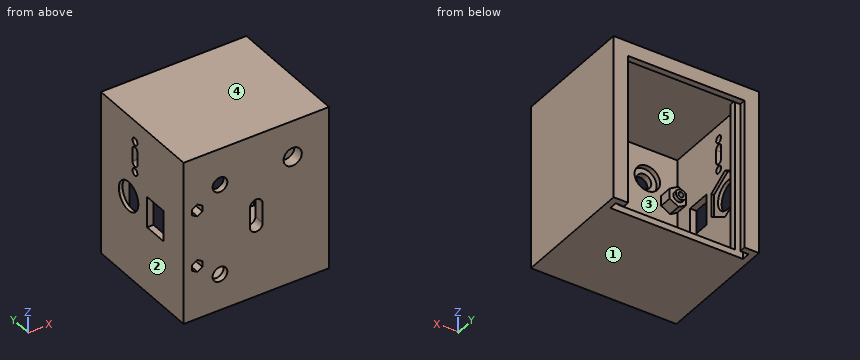
from build123d import *

# Parameters (mm, degrees)
SKETCH1_W               = 80
SKETCH1_H               = 90
BOSS_EXTRUDE1_DEPTH     = 6
SKETCH4_W               = 80
SKETCH4_H               = 90
SKETCH4_W_2             = 73
SKETCH4_H_2             = 83
BOSS_EXTRUDE2_DEPTH     = 54
SKETCH6_R               = 4.05
SKETCH6_R_2             = 5
CUT_EXTRUDE1_DEPTH      = 40
SKETCH7_R               = 7
CUT_EXTRUDE2_DEPTH      = 2.8
BOSS_EXTRUDE3_DEPTH     = 7
SKETCH11_R              = 2.85
BOSS_EXTRUDE4_DEPTH     = 2
CUT_EXTRUDE3_DEPTH      = 9
CUT_EXTRUDE3_DEPTH_BACK = 6
SKETCH5_R               = 1.5
CUT_EXTRUDE4_DEPTH      = 6
CUT_EXTRUDE4_DEPTH_BACK = 81.876448982
SKETCH12_W              = 17
SKETCH12_H              = 13.5
CUT_EXTRUDE6_DEPTH      = 3.5
SKETCH17_R              = 8
CUT_EXTRUDE8_DEPTH      = 2
CUT_EXTRUDE9_DEPTH      = 1.5
CUT_EXTRUDE10_DEPTH     = 10
BOSS_EXTRUDE5_DEPTH     = 90
BOSS_EXTRUDE5_2_DEPTH   = 90
SKETCH21_W              = 3.5
SKETCH21_H              = 8
BOSS_EXTRUDE6_DEPTH     = 80
SKETCH22_W              = 80
SKETCH22_H              = 3.5
BOSS_EXTRUDE7_DEPTH     = 4.5
SKETCH24_W              = 8
SKETCH24_H              = 3.5
BOSS_EXTRUDE8_DEPTH     = 90
SKETCH26_R              = 2
CUT_EXTRUDE11_DEPTH     = 3.5


with BuildPart() as part:
    # Sketch1 → Boss-Extrude1 (new body)
    with BuildSketch(Plane(origin=(0, 0, 0), x_dir=(1, 0, 0), z_dir=(0, 1, 0))):
        Rectangle(SKETCH1_W, SKETCH1_H)
    extrude(amount=BOSS_EXTRUDE1_DEPTH)

    # Sketch4 → Boss-Extrude2 (add)
    with BuildSketch(Plane(origin=(0, 6, 0), x_dir=(1, 0, 0), z_dir=(0, 1, 0))):
        Rectangle(SKETCH4_W, SKETCH4_H)
        Rectangle(SKETCH4_W_2, SKETCH4_H_2, mode=Mode.SUBTRACT)
    extrude(amount=BOSS_EXTRUDE2_DEPTH)

    # Sketch6 → Cut-Extrude1 (cut)
    with BuildSketch(Plane(origin=(0, 6, 0), x_dir=(1, 0, 0), z_dir=(0, 1, 0))):
        with Locations(Location((-20, 25, 0), (0, 0, 270))):
            Circle(SKETCH6_R)
        with Locations(Location((-20, -25, 0), (0, 0, 270))):
            Circle(SKETCH6_R)
        with Locations(Location((20, -25, 0), (0, 0, 270))):
            Circle(SKETCH6_R_2)
    extrude(amount=-CUT_EXTRUDE1_DEPTH, mode=Mode.SUBTRACT)

    # Sketch7 → Cut-Extrude2 (cut)
    with BuildSketch(Plane(origin=(0, 6, 0), x_dir=(1, 0, 0), z_dir=(0, 1, 0))):
        with Locations(Location((-20, 25, 0), (0, 0, 270))):
            Circle(SKETCH7_R)
        with Locations(Location((-20, -25, 0), (0, 0, 270))):
            Circle(SKETCH7_R)
    extrude(amount=-CUT_EXTRUDE2_DEPTH, mode=Mode.SUBTRACT)

    # Sketch10 → Boss-Extrude3 (add)
    with BuildSketch(Plane(origin=(0, 6, 0), x_dir=(1, 0, 0), z_dir=(0, 1, 0))):
        Polygon((-32.5, 21.100297611), (-37.35, 18.300148806), (-37.35, 12.699851194), (-32.5, 9.899702389), (-27.65, 12.699851194), (-27.65, 18.300148806), align=None)
        Polygon((-27.65, -12.699851194), (-32.5, -9.899702389), (-37.35, -12.699851194), (-37.35, -18.300148806), (-32.5, -21.100297611), (-27.65, -18.300148806), align=None)
    extrude(amount=BOSS_EXTRUDE3_DEPTH)

    # Sketch11 → Boss-Extrude4 (add)
    with BuildSketch(Plane(origin=(0, 13, 0), x_dir=(1, 0, 0), z_dir=(0, 1, 0))):
        with Locations(Location((-32.5, 15.5, 0), (0, 0, 270))):
            Circle(SKETCH11_R)
        with Locations(Location((-32.5, -15.5, 0), (0, 0, 270))):
            Circle(SKETCH11_R)
    extrude(amount=BOSS_EXTRUDE4_DEPTH)

    # Sketch5 → Cut-Extrude3 (cut, two sides: drawn at the far end of the back side and taken through both)
    with BuildSketch(Plane(origin=(0, 6, 0), x_dir=(1, 0, 0), z_dir=(0, 1, 0)).offset(-CUT_EXTRUDE3_DEPTH_BACK)):
        with Locations(Location((-32.5, 15.5, 0), (0, 0, 270))):
            Circle(SKETCH5_R)
        with Locations(Location((-32.5, -15.5, 0), (0, 0, 270))):
            Circle(SKETCH5_R)
    extrude(amount=CUT_EXTRUDE3_DEPTH + CUT_EXTRUDE3_DEPTH_BACK, mode=Mode.SUBTRACT)

    # Sketch8 → Cut-Extrude4 (cut, two sides: drawn at the far end of the back side and taken through both)
    with BuildSketch(Plane(origin=(0, 6, 0), x_dir=(1, 0, 0), z_dir=(0, 1, 0)).offset(-CUT_EXTRUDE4_DEPTH_BACK)):
        Polygon((-29.65, 17.145448267), (-32.5, 18.790896534), (-35.35, 17.145448267), (-35.35, 13.854551733), (-32.5, 12.209103466), (-29.65, 13.854551733), align=None)
        Polygon((-29.65, -13.854551733), (-32.5, -12.209103466), (-35.35, -13.854551733), (-35.35, -17.145448267), (-32.5, -18.790896534), (-29.65, -17.145448267), align=None)
    extrude(amount=CUT_EXTRUDE4_DEPTH + CUT_EXTRUDE4_DEPTH_BACK, mode=Mode.SUBTRACT)

    # Sketch12 → Cut-Extrude6 (cut)
    with BuildSketch(Plane(origin=(-36.5, 0, 0), x_dir=(0, 0, -1), z_dir=(1, 0, 0))):
        with Locations((0, 23.25)):
            Rectangle(SKETCH12_W, SKETCH12_H)
    extrude(amount=-CUT_EXTRUDE6_DEPTH, mode=Mode.SUBTRACT)

    # Sketch17 → Cut-Extrude8 (cut)
    with BuildSketch(Plane.ZY.offset(40)):
        with Locations((0, 45.25)):
            Circle(SKETCH17_R)
    extrude(amount=-CUT_EXTRUDE8_DEPTH, mode=Mode.SUBTRACT)

    # Sketch15 → Cut-Extrude9 (cut)
    with BuildSketch(Plane(origin=(-36.5, 0, 0), x_dir=(0, 0, -1), z_dir=(1, 0, 0))):
        Polygon((-6.495190528, 56.5), (-12.990381057, 45.25), (-6.495190528, 34), (6.495190528, 34), (12.990381057, 45.25), (6.495190528, 56.5), align=None)
    extrude(amount=-CUT_EXTRUDE9_DEPTH, mode=Mode.SUBTRACT)

    # Sketch19 → Cut-Extrude10 (cut)
    with BuildSketch(Plane(origin=(0, 6, 0), x_dir=(1, 0, 0), z_dir=(0, 1, 0))):
        with BuildLine():
            Line((-3.5, -5.5), (-3.5, 5.5))
            ThreePointArc((-3.5, 5.5), (0, 9), (3.5, 5.5))
            Line((3.5, 5.5), (3.5, -5.5))
            ThreePointArc((3.5, -5.5), (0, -9), (-3.5, -5.5))
        make_face()
    extrude(amount=-CUT_EXTRUDE10_DEPTH, mode=Mode.SUBTRACT)



with BuildPart() as body_2:
    # Sketch20 → Boss-Extrude5 (new body)
    with BuildSketch(Plane(origin=(0, 0, -45), x_dir=(-1, 0, 0), z_dir=(0, 0, -1))):
        Polygon((-40, 60), (-36.5, 60), (-36.5, 64.5), (-32, 64.5), (-32, 68), (-40, 68), align=None)
    extrude(amount=-BOSS_EXTRUDE5_DEPTH)


with BuildPart() as body_3:
    # Sketch20 → Boss-Extrude5 2 (new body)
    with BuildSketch(Plane(origin=(0, 0, -45), x_dir=(-1, 0, 0), z_dir=(0, 0, -1))):
        Polygon((40, 60), (36.5, 60), (36.5, 64.5), (32, 64.5), (32, 68), (40, 68), align=None)
    extrude(amount=-BOSS_EXTRUDE5_2_DEPTH)


with BuildPart() as part_1:
    add(part.part)

    add(body_2.part)  # Boss-Extrude6 merges body 2
    # Sketch21 → Boss-Extrude6 (add)
    with BuildSketch(Plane(origin=(40, 0, 0), x_dir=(0, 0, -1), z_dir=(1, 0, 0))):
        with Locations((-43.25, 64)):
            Rectangle(SKETCH21_W, SKETCH21_H)
    extrude(amount=-BOSS_EXTRUDE6_DEPTH)


    add(body_3.part)  # Boss-Extrude7 merges body 3
    # Sketch22 → Boss-Extrude7 (add)
    with BuildSketch(Plane(origin=(0, 0, 41.5), x_dir=(-1, 0, 0), z_dir=(0, 0, -1))):
        with Locations((0, 66.25)):
            Rectangle(SKETCH22_W, SKETCH22_H)
    extrude(amount=BOSS_EXTRUDE7_DEPTH)

    # Sketch24 → Boss-Extrude8 (add)
    with BuildSketch(Plane.XY.offset(45)):
        with Locations((-36, 58.25)):
            Rectangle(SKETCH24_W, SKETCH24_H)
        with Locations((36, 58.25)):
            Rectangle(SKETCH24_W, SKETCH24_H)
    extrude(amount=-BOSS_EXTRUDE8_DEPTH)

    # Sketch26 → Cut-Extrude11 (cut)
    with BuildSketch(Plane.ZY.offset(40)):
        with Locations((16.5, 40)):
            Circle(SKETCH26_R)
        with Locations((33.5, 40)):
            Circle(SKETCH26_R)
        with BuildLine():
            Line((21.5, 42), (28.5, 42))
            ThreePointArc((28.5, 42), (30.5, 40), (28.5, 38))
            Line((28.5, 38), (21.5, 38))
            ThreePointArc((21.5, 38), (19.5, 40), (21.5, 42))
        make_face()
    extrude(amount=-CUT_EXTRUDE11_DEPTH, mode=Mode.SUBTRACT)


solid = part_1.part
Can you work these out from the model? Positions are in its coordinate system, mm. Face numbers are marked on the shaded views. A direction names the side the tool comes from. Give positions to 0.01 mm unless a question says otherwise; leave off trailing zeros. Write each loop counter-clockwise with the first axis right and the second up, starting at its lowest first coordinate (ties: lowest second). Pieces come first, ordered by that corner, then holes. Notation, with made-up numbers: M 20,-19 L 33,-19 A35 cw 33,13 Z; hole C 11,-14 d11. An arc over 180 degrees is marked long. Answer in a Markdown table with one row per item. Add a question column.
Item 1: Imagine slicing it at C-C, the plane y = 10.5. State how many separate pieces and enclosed holes the cut face has, plus the area to 3 significant figures.
Item 2: We'd pull the mould along X, two halves only. Please class the marked faces 1, 2 and 3: released by +X, released by -X, zero draft, split by the parting line, or undercut.
Item 3: Please list where these lines run through material, in increasing order: L1, parallel to X at y = 12.8, z = -15.5; L2, parallel to X at y = 2.45, z = 25; L3, parallel to Z at x = -23, y = 38.
Item 4: Imagine slicing it at D-D, the plane x = 0. Write out the boundary of the cut face in (y, z), plus the area to 3 significant figures.
Item 5: For pin 1 Ø5 at (x, z) = (25.5, 2) entering from +Y; pin 2 Ø3 at (x, z) = (-21.5, 24) entering from +Y; pin 3 Ø3.5 at (y, z) = (40, 16.5) entering from -X, each with a flat end and sliding along its axis, tell me the tip position at first contact or that it passes through.
Item 6: Imagine slicing it at A-A, the plane x = -20. Write out the boundary of the cut face in (y, z), plus the area to 3 significant figures.
Item 7: On a 3-axis mill with a long thin cutter (end or side, diameter ignored), from which of +Z, -Z, +X, -X, +Y, -Y can I reach the whole of each face in a straight line? I mean the marked faces 4 and 5. Say none if no direction works.
Evaluation:
| question | item | result |
|---|---|---|
| 1 | separate pieces | 1 |
| 1 | enclosed holes | 3 |
| 1 | area | 1,240 mm² |
| 2 | face 1 | zero draft |
| 2 | face 2 | released by -X |
| 2 | face 3 | undercut |
| 3 | L1 | x = -40 to -34, -31 to -27.65, 36.5 to 40 |
| 3 | L2 | x = -40 to -24.05, -15.95 to 15, 25 to 40 |
| 3 | L3 | z = -45 to -41.5, 41.5 to 45 |
| 4 | outline | M 0,-45 L 60,-45 L 60,-41.5 L 6,-41.5 L 6,-9 L 0,-9 Z; M 0,9 L 6,9 L 6,41.5 L 64.5,41.5 L 64.5,37 L 68,37 L 68,45 L 0,45 Z |
| 4 | area | 854 mm² |
| 5 | pin 1 | stops at y = 6 |
| 5 | pin 2 | passes through |
| 5 | pin 3 | stops at x = 36.5 |
| 6 | outline | M 0,-45 L 60,-45 L 60,-41.5 L 6,-41.5 L 6,-32 L 3.2,-32 L 3.2,-29.05 L 0,-29.05 Z; M 0,-20.95 L 3.2,-20.95 L 3.2,-18 L 6,-18 L 6,18 L 3.2,18 L 3.2,20.95 L 0,20.95 Z; M 0,29.05 L 3.2,29.05 L 3.2,32 L 6,32 L 6,41.5 L 64.5,41.5 L 64.5,37 L 68,37 L 68,45 L 0,45 Z |
| 6 | area | 832 mm² |
| 7 | face 4 | +Z, +X, -X, +Y, -Y |
| 7 | face 5 | none |
